Here's how the part is built. I have some questions about the finished solid (model axes, mm). Face numbers are marked on the shaded views. Coordinates: 2 decimals unless noted, no trailing zeros. Write each loop counter-clockwise with the first axis right and the second up, starting at its lowest first coordinate (ties: lowest second). Pieces come first, ordered by that corner, then holes. Notation, with made-up numbers: (45.25, 33) -> (74.25, 33) arc R27 ccw to (74.25, 54) -> close; hole circle Ø11 at (47.5, 57). An arc over 180 degrees is marked (long way). Put each result on its own line as item: value.
```python
from build123d import *

# Parameters (mm, degrees)
SKETCH1_W           = 7.5
SKETCH1_H           = 10
BOSS_EXTRUDE1_DEPTH = 7.5
SKETCH2_R           = 2.5
CUT_EXTRUDE1_DEPTH  = 7.5
SKETCH3_W           = 10
SKETCH3_H           = 1
CUT_EXTRUDE2_DEPTH  = 0.5


with BuildPart() as part:
    # Sketch1 → Boss-Extrude1 (new body)
    with BuildSketch(Plane(origin=(0, 0, 0), x_dir=(0, 1, 0), z_dir=(0, 0, 1))):
        with Locations((-0.026595745, -0.292553191)):
            Rectangle(SKETCH1_W, SKETCH1_H)
    extrude(amount=BOSS_EXTRUDE1_DEPTH)

    # Sketch2 → Cut-Extrude1 (cut)
    with BuildSketch(Plane.XY.offset(7.5)):
        with Locations((-0.707446809, 0)):
            Circle(SKETCH2_R)
    extrude(amount=-CUT_EXTRUDE1_DEPTH, mode=Mode.SUBTRACT)

    # Sketch3 → Cut-Extrude2 (cut)
    with BuildSketch(Plane(origin=(0, 0, 0), x_dir=(1, 0, 0), z_dir=(0, 0, -1))):
        with Locations((0.292553191, 1.526595745)):
            Rectangle(SKETCH3_W, SKETCH3_H)
        with Locations((0.292553191, -1.473404255)):
            Rectangle(SKETCH3_W, SKETCH3_H)
    extrude(amount=-CUT_EXTRUDE2_DEPTH, mode=Mode.SUBTRACT)


solid = part.part
```
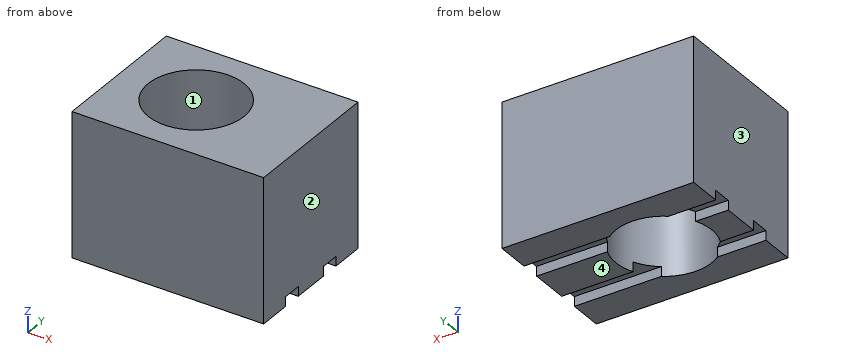
Item 1: Imagine slicing it at A-A on y = 0. Write out the boundary of the cut face in (x, z).
Output:
outline: (-4.71, 0) -> (-3.21, 0) -> (-3.21, 7.5) -> (-4.71, 7.5) -> close; (1.79, 0) -> (5.29, 0) -> (5.29, 7.5) -> (1.79, 7.5) -> close
Item 2: For P1, Ø4, axis at x = 1.5, y = -1.5, coming from the -Z side; P2, Ø4.5, axis at x = -0.71, y = 0, coming from the -Z side; P3, Ø0.8, axis at x = 3.5, y = 1.5, coming from the -Z side, each with a flat end and sliding along its axis, tell me the tip position at first contact or that it passes through.
Output:
P1: stops at z = 0
P2: passes through
P3: stops at z = 0.5
Item 3: If we mould it in two halves opening along X, with no side actions, what happens to the marked faces 1, 2, 3 and 4? For each: released by +X, released by -X, zero draft, split by the parting line, or undercut.
Output:
face 1: undercut
face 2: released by +X
face 3: released by -X
face 4: zero draft
Item 4: Imagine slicing it at D-D on x = -4. Write out the boundary of the cut face in (y, z), then the cut area to 4 significant figures.
Output:
outline: (-3.78, 0) -> (-2.03, 0) -> (-2.03, 0.5) -> (-1.03, 0.5) -> (-1.03, 0) -> (0.97, 0) -> (0.97, 0.5) -> (1.97, 0.5) -> (1.97, 0) -> (3.72, 0) -> (3.72, 7.5) -> (-3.78, 7.5) -> close
area: 55.25 mm²
Item 5: Imagine slicing it at C-C on x = 0.5. Write out the boundary of the cut face in (y, z).
Output:
outline: (-3.78, 0) -> (-2.19, 0) -> (-2.19, 7.5) -> (-3.78, 7.5) -> close; (2.19, 0) -> (3.72, 0) -> (3.72, 7.5) -> (2.19, 7.5) -> close
Item 6: Please list where these lines run through material, in increasing order: line 1 along X through (y, z) = (0, 4.5); line 2 along Z through (x, y) = (2.5, -1.5); line 3 along Y through (x, z) = (0, 3.75). Write a range as from..to.
Output:
line 1: x = -4.71..-3.21, 1.79..5.29
line 2: z = 0.5..7.5
line 3: y = -3.78..-2.4, 2.4..3.72
Item 7: Imagine slicing it at B-B on z = 1.5. Write out the boundary of the cut face in (x, y).
Output:
outline: (-4.71, -3.78) -> (5.29, -3.78) -> (5.29, 3.72) -> (-4.71, 3.72) -> close; hole circle Ø5 at (-0.71, 0)
